```python
from build123d import *

# Parameters (mm, degrees)
SKETCH1_W           = 25.4
SKETCH1_H           = 15.24
BOSS_EXTRUDE1_DEPTH = 3.175
SKETCH3_R           = 4.761366165
SKETCH3_R_2         = 1.5875
BOSS_EXTRUDE2_DEPTH = 15.24


with BuildPart() as part:
    # Sketch1 → Boss-Extrude1 (new body)
    with BuildSketch(Plane(origin=(0, 0, 0), x_dir=(1, 0, 0), z_dir=(0, 1, 0))):
        with Locations((-33.04393404, -21.504734982)):
            Rectangle(SKETCH1_W, SKETCH1_H)
    extrude(amount=BOSS_EXTRUDE1_DEPTH)

    # Sketch3 → Boss-Extrude2 (add)
    with BuildSketch(Plane.XY.offset(29.124734982)):
        with Locations((-45.670474152, 4.76079945)):
            Circle(SKETCH3_R)
        with Locations((-45.670474152, 4.76079945)):
            Circle(SKETCH3_R_2, mode=Mode.SUBTRACT)
    extrude(amount=-BOSS_EXTRUDE2_DEPTH)


solid = part.part
```
Source: CAD feature listing. Evaluate the final solid. Frame: model axes, mm. Round coordinates to 2 decimals unless told otherwise and drop trailing zeros. Order: outer loops, then holes, each group sorted by start corner. A loop starts at its lowest first (then second) coordinate and runs counter-clockwise, first axis right, second up. Notation, with made-up numbers: (27.25, 68) -> (51.25, 68) arc R22 cw to (51.25, 91) -> close; hole circle Ø1 at (-38, -23.5). An arc over 180 degrees is marked (long way). One line per item, written item: value. Start each with the question number.
Q1. Material intervals for probe 1 along Y at (x, z) = (-34.5, 22) (3 decimals); probe 2 along X at (y, z) = (6, 23); probe 3 along X at (y, z) = (4.25, 18), sorted ascending.
Q2. Section query D-D (y = 4). Return the cut outline in (x, z), plus the area to 3 significant figures.
Q3. Pin query (flat end, axial travel): pin 1 (1.5 mm diameter, centred on y = 7.5, z = 24, fed in from -X); pin 2 (3 mm diameter, centred on x = -24, z = 21, fed in from +Y) (3 decimals). Return the tip coordinate at first contact, or that it passes through.
Q4. Section query C-C (x = -34.5). Return the cut outline in (y, z) (3 decimals), plus the area to 3 significant figures.
Q5. Section query B-B (y = 6). Return the cut outline in (x, z), plus the area to 3 significant figures.
Findings below:
1. probe 1: 0 to 3.175
1. probe 2: -50.27 to -46.66, -44.68 to -41.07
1. probe 3: -50.4 to -47.17, -44.17 to -40.94
2. outline: (-50.37, 13.88) -> (-47.06, 13.88) -> (-47.06, 29.12) -> (-50.37, 29.12) -> close; (-44.28, 13.88) -> (-40.97, 13.88) -> (-40.97, 29.12) -> (-44.28, 29.12) -> close
2. area: 101 mm²
3. pin 1: x = -50
3. pin 2: y = 3.175
4. outline: (0, 13.885) -> (3.175, 13.885) -> (3.175, 29.125) -> (0, 29.125) -> close
4. area: 48.4 mm²
5. outline: (-50.27, 13.88) -> (-46.66, 13.88) -> (-46.66, 29.12) -> (-50.27, 29.12) -> close; (-44.68, 13.88) -> (-41.07, 13.88) -> (-41.07, 29.12) -> (-44.68, 29.12) -> close
5. area: 110 mm²
